Could you check a few things on this drawing? It's one solid part, dimensions in mm from its lowest x, y, z. Round coordinates to 2 decimals unless told otherwise and drop trailing zeros. Write each loop counter-clockwise with the first axis right and the second up, starting at its lowest first coordinate (ties: lowest second). Pieces come first, ordered by that corner, then holes. Notation, with made-up numbers: M -19,-34.75 L 31,-34.75 A13 ccw 31,-29.75 Z; hole C 59,39.5 d1. An arc over 180 degrees is marked long. One line per item, written item: value. Start each with the question number.
(1) If I drill on L1, parallel to Y at x = 25, z = 2.9; L2, parallel to X at y = 42.5, z = 4.5; L3, parallel to Z at x = 39.5, y = 12.5, over which ranges is the centre line in solid material (lowest first)?
(2) Thinking about a two-plate mould opening in X: for the marked faces 1, 2 and 3, which applies, released by +X, released by -X, zero draft, split by the parting line, or undercut?
(3) I'm going to push flat-ended pins straight in: pin 1 Ø2 at (x, y) = (28.5, 22.5) entering from -Z; pin 2 Ø2 at (y, z) = (43.5, 4.5) entering from -X; pin 3 Ø1 at (x, z) = (20, 5.5) entering from -Y. Where does each tip first touch, or does it pass through?
(4) I want a section at C-C on z = 2.75. Please give me the cut outline in (x, y).
(5) I want a section at A-A on y = 25. Please give me the cut outline in (x, z), and give its area (4 significant figures).
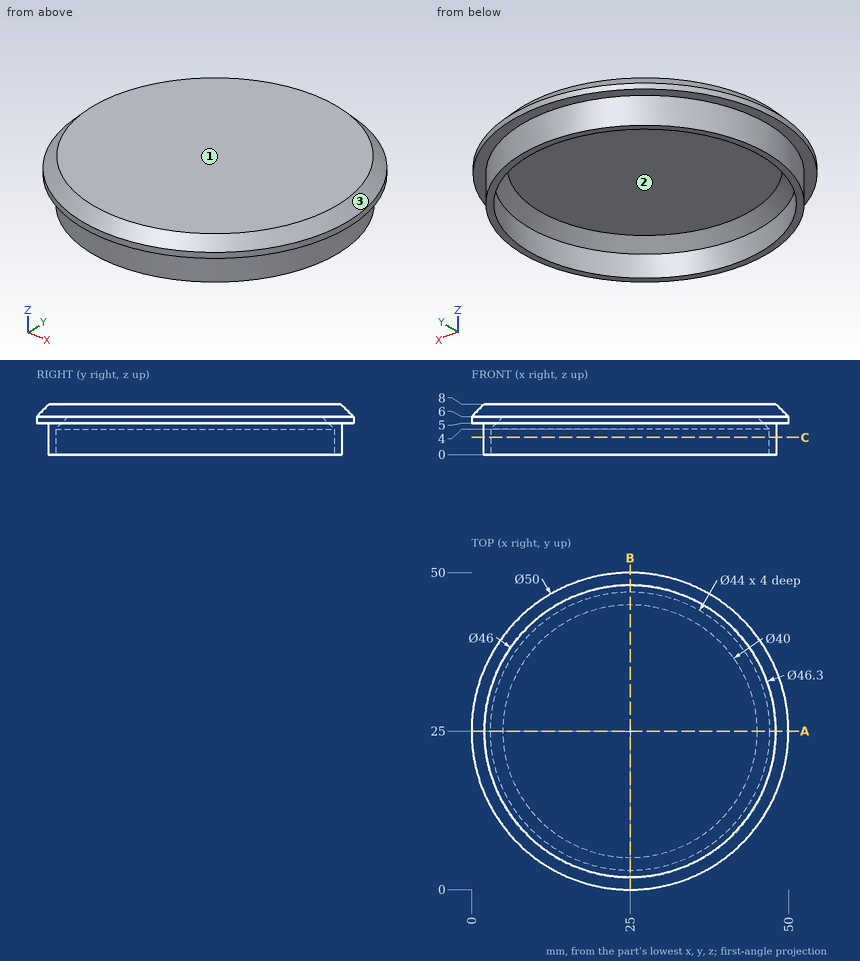
Found:
1. L1: y = 1.85 to 3, 47 to 48.15
1. L2: x = 9.85 to 12.51, 37.49 to 40.15
1. L3: z = 6 to 8
2. face 1: zero draft
2. face 2: undercut
2. face 3: split by the parting line
3. pin 1: stops at z = 6
3. pin 2: stops at x = 7.28
3. pin 3: stops at y = 0.41
4. outline: C 25,25 d46.3; hole C 25,25 d44
5. outline: M 0,5 L 1.85,5 L 1.85,0 L 3,0 L 3,4 L 5,6 L 45,6 L 47,4 L 47,0 L 48.15,0 L 48.15,5 L 50,5 L 50,6 L 48,8 L 2,8 L 0,6 Z
5. area: 117.5 mm²
